CAD build for the part. Positions are in the model's coordinates, mm. Round coordinates to 2 decimals unless told otherwise and drop trailing zeros. Order: outer loops, then holes, each group sorted by start corner. A loop starts at its lowest first (then second) coordinate and runs counter-clockwise, first axis right, second up. Notation, with made-up numbers: M -18.75,11 L 7.25,11 A24 cw 7.25,48 Z; hole C 10,-5.5 d6. An arc over 180 degrees is marked long. Answer as a JSON object with one key per item and string values.
Autodesk Fusion 360 part; units mm, degrees
sketch "Sketch1" plane through (0, 0, 0) normal (0, 0, 1) x (1, 0, 0)
  line L0 (6.508, 15) -> (-6.508, 15)
  line L1 (-6.508, 15) -> (-6.508, -15)
  line L2 (-6.508, -15) -> (6.508, -15)
  line L3 (6.508, -15) -> (6.508, 15)
  line L4 (6.508, 15) -> (-6.508, -15) construction
  line L5 (-6.508, 15) -> (6.508, -15) construction
  line L6 (0, 15) -> (0, -15) construction
  circle A0 centre (0, 13) radius 2
  circle A1 centre (0, 9.5) radius 1.5
  circle A2 centre (0, 6) radius 2
  circle A3 centre (0, 2.5) radius 1.5
  circle A4 centre (0, -1) radius 2
  circle A5 centre (0, -4.5) radius 1.5
  circle A6 centre (0, -8) radius 2
  circle A7 centre (0, -11.5) radius 1.5
  dimension "d1" = 13.016
  dimension "d2" = 30
  dimension "d3" = 4
  dimension "d4" = 3
  dimension "d5" = 4
  dimension "d6" = 3
  dimension "d7" = 4
  dimension "d8" = 3
  dimension "d9" = 4
  dimension "d10" = 3
extrude "Extrude1" add sketch "Sketch1" along normal blind 0.5 contours A6 | A4 | A2 | A0 | L0 L1 L2 L3
Item 1: Saw through at A-A on z = 0.3. List the corners of the cut face in (x, y).
Worked answers:
{"outline": "M -6.51,-15 L 6.51,-15 L 6.51,15 L -6.51,15 Z; hole C 0,-11.5 d3; hole C 0,-4.5 d3; hole C 0,2.5 d3; hole C 0,9.5 d3"}
Item 2: Saw through at C-C on y = -11.5. List the corners of the cut face in (x, z).
Worked answers:
{"outline": "M -6.51,0 L -1.5,0 L -1.5,0.5 L -6.51,0.5 Z; M 1.5,0 L 6.51,0 L 6.51,0.5 L 1.5,0.5 Z"}
Item 3: Saw through at B-B on x = 0. List the corners of the cut face in (y, z), and give its area (3 significant figures).
Worked answers:
{"outline": "M -15,0 L -13,0 L -13,0.5 L -15,0.5 Z; M -10,0 L -6,0 L -6,0.5 L -10,0.5 Z; M -3,0 L 1,0 L 1,0.5 L -3,0.5 Z; M 4,0 L 8,0 L 8,0.5 L 4,0.5 Z; M 11,0 L 15,0 L 15,0.5 L 11,0.5 Z", "area": "9.00 mm2"}
Item 4: Two-plate mould, pull along Y, no slides. Class faces 1 (the flat face through (0, 0, 0.5)), 2 (the cylindrical face through (-0.325, -10.036, 0.246)): released by +Y, released by -Y, zero draft, split by the parting line, or undercut.
Worked answers:
{"face 1": "zero draft", "face 2": "undercut"}
Item 5: Wall check: line 1 along Y through (x, z) = (0, 0.4); line 2 along Y through (x, z) = (-1, 0.3); line 3 along X through (y, z) = (-5.75, 0.35). Give the ranges that are in metal, low to high. Write a range as [from, to].
Worked answers:
{"line 1": "y = [-15, -13], [-10, -6], [-3, 1], [4, 8], [11, 15]", "line 2": "y = [-15, -12.62], [-10.38, -5.62], [-3.38, 1.38], [3.62, 8.38], [10.62, 15]", "line 3": "x = [-6.51, -0.83], [0.83, 6.51]"}
